Could you check a few things on this drawing? It's one solid part, dimensions in mm from its lowest x, y, z. A direction names the side the tool comes from. Round coordinates to 2 decimals unless told otherwise and drop trailing zeros. Loops run counter-clockwise (first coordinate to the right, second up) from the corner with the lowest first, then second, coordinate; pieces in that order, holes last. Notation, with made-up numbers: (57.5, 48) -> (93.5, 48) arc R21 cw to (93.5, 68) -> close; hole circle Ø2 at (-11, 49.5). An arc over 180 degrees is marked (long way). Use one line per item in the form item = value. Start each with the question number.
Item 1: If I drill on L1, parallel to Y at x = 78.5, z = 27; L2, parallel to Z at x = 26.5, y = 54 (1 decimal); L3, parallel to Z at x = 36, y = 46 (1 decimal), over which ranges is the centre line in solid material (lowest first)? Write a range as [from, to].
Item 2: If we section it at C-C (x = 45.5): Write out the boundary of the cut face in (y, z) (1 decimal), then the cut area to 3 significant figures.
Item 3: For the marked faces 4, 5 and 6, which set-ups out of +Z, -Z, +X, -X, +Y, -Y let a thin tool reach every point of the face, with its end or its side?
Item 4: If we section it at D-D (y = 81.5): Write out the boundary of the cut face in (x, z).
Item 5: If we section it at B-B (y = 47): Write out the boundary of the cut face in (x, z) (1 decimal).
Item 6: I'm going to push a flat-ended pin straight in: pin 1 Ø6 at (x, z) = (35, 93) entering from -Y. Where does the tip first touch, or does it pass through?
Item 7: Thinking about a two-plate mould opening in Z: for the marked faces 1, 2 and 3, which applies, released by +Z, released by -Z, zero draft, split by the parting line, or undercut?
Item 8: If we section it at A-A (z = 48.5): Write out the boundary of the cut face in (x, y).
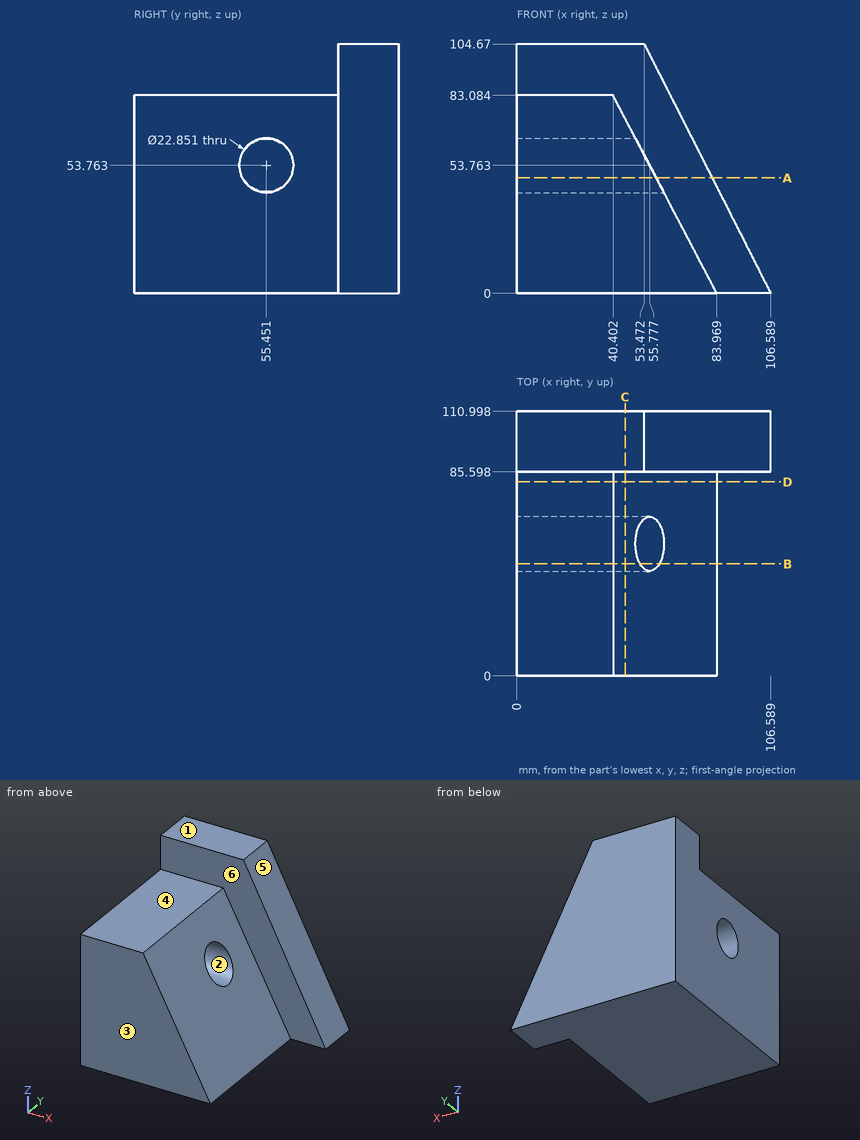
Values found:
q1.L1 = [85.6, 111]
q1.L2 = [0, 42.4], [65.1, 83.1]
q1.L3 = [0, 47.3], [60.2, 83.1]
q2.outline = (0, 0) -> (111, 0) -> (111, 104.7) -> (85.6, 104.7) -> (85.6, 73.4) -> (0, 73.4) -> close; hole circle Ø22.9 at (55.5, 53.8)
q2.area = 8,530 mm2
q3.face_4 = +Z, +X, -X, -Y
q3.face_5 = +Z, +X, +Y, -Y
q3.face_6 = +Z, +X, -Y
q4.outline = (0, 0) -> (83.97, 0) -> (40.4, 83.08) -> (0, 83.08) -> close
q5.outline = (0, 0) -> (84, 0) -> (59.8, 46.1) -> (0, 46.1) -> close; (0, 61.5) -> (51.7, 61.5) -> (40.4, 83.1) -> (0, 83.1) -> close
q6.pin_1 = 85.6
q7.face_1 = released by +Z
q7.face_2 = undercut
q7.face_3 = zero draft
q8.outline = (0, 0) -> (58.54, 0) -> (58.54, 45.31) -> (0, 45.31) -> close; (0, 65.59) -> (58.54, 65.59) -> (58.54, 85.6) -> (81.98, 85.6) -> (81.98, 111) -> (0, 111) -> close
